```python
from build123d import *

# Parameters (mm, degrees)
SKETCH1_W                      = 15.24
SKETCH1_H                      = 15.24
BASE_FLANGE1_DEPTH             = 1.5875
EDGE_FLANGE1_STRIP_W           = 8.228
EDGE_FLANGE1_STRIP_H           = 1.5875
EDGE_FLANGE1_STRIP_CUT_DEPTH   = 15.24
EDGE_FLANGE1_STRIP_2_W         = 8.228
EDGE_FLANGE1_STRIP_2_H         = 1.5875
EDGE_FLANGE1_STRIP_CUT_2_DEPTH = 15.24
EDGE_FLANGE1_DEPTH             = 15.24
EDGE_FLANGE1_BEND_DEPTH        = 15.24
CUT_EXTRUDE2_REACH             = 30.592
CUT_EXTRUDE1_REACH             = 30.592
SKETCH13_R                     = 3.2639


# Sheet-metal steps are written as plain solids
with BuildPart() as part:
    # Sketch1 → Base-Flange1 (new body)
    with BuildSketch(Plane(origin=(0, 0, 0), x_dir=(1, 0, 0), z_dir=(0, 1, 0))):
        Rectangle(SKETCH1_W, SKETCH1_H)
    extrude(amount=-BASE_FLANGE1_DEPTH)

    # Edge-Flange1 strip (across the edge) → Edge-Flange1 strip cut (cut)
    with BuildSketch(Plane(origin=(-7.72, 0, -7.62), x_dir=(1, 0, 0), z_dir=(0, 0, 1))):
        with Locations((-3.225, -0.79375)):
            Rectangle(EDGE_FLANGE1_STRIP_W, EDGE_FLANGE1_STRIP_H)
    extrude(amount=EDGE_FLANGE1_STRIP_CUT_DEPTH, mode=Mode.SUBTRACT)

    # Edge-Flange1 strip 2 (across the edge) → Edge-Flange1 strip cut 2 (cut)
    with BuildSketch(Plane(origin=(7.72, 0, 7.62), x_dir=(-1, 0, 0), z_dir=(0, 0, -1))):
        with Locations((-3.225, -0.79375)):
            Rectangle(EDGE_FLANGE1_STRIP_2_W, EDGE_FLANGE1_STRIP_2_H)
    extrude(amount=EDGE_FLANGE1_STRIP_CUT_2_DEPTH, mode=Mode.SUBTRACT)

    # Edge-Flange1 section (across the edge) → Edge-Flange1 (add)
    with BuildSketch(Plane(origin=(-7.72, 0, -7.62), x_dir=(1, 0, 0), z_dir=(0, 0, 1))):
        with BuildLine():
            Line((-1.5875, 0.889), (-1.5875, 20.32))
            Line((-1.5875, 20.32), (0, 20.32))
            Line((0, 20.32), (0, 0.889))
            ThreePointArc((0, 0.889), (0.260382072, 0.260382072), (0.889, 0))
            Line((0.889, 0), (0.889, -1.5875))
            ThreePointArc((0.889, -1.5875), (-0.862149944, -0.862149944), (-1.5875, 0.889))
        make_face()
    extrude(amount=EDGE_FLANGE1_DEPTH)

    # Edge-Flange1 section 2 (across the edge) → Edge-Flange1 bend (add)
    with BuildSketch(Plane(origin=(7.72, 0, 7.62), x_dir=(-1, 0, 0), z_dir=(0, 0, -1))):
        with BuildLine():
            Line((-1.5875, 0.889), (-1.5875, 20.32))
            Line((-1.5875, 20.32), (0, 20.32))
            Line((0, 20.32), (0, 0.889))
            ThreePointArc((0, 0.889), (0.260382072, 0.260382072), (0.889, 0))
            Line((0.889, 0), (0.889, -1.5875))
            ThreePointArc((0.889, -1.5875), (-0.862149944, -0.862149944), (-1.5875, 0.889))
        make_face()
    extrude(amount=EDGE_FLANGE1_BEND_DEPTH)

    # Cut-Extrude2: up to this face of the body (flat: up to its plane)
    cut_extrude2_end = Plane(part.part.faces().sort_by_distance((9.3075, 10.6045, 0))[0])
    # Sketch14 → Cut-Extrude2 (cut, up to the picked face)
    with BuildSketch(Plane.ZY.offset(9.3075), mode=Mode.PRIVATE) as cut_extrude2_sk1:
        with BuildLine():
            Line((-7.62, 20.32), (-7.62, 12.7))
            ThreePointArc((-7.62, 12.7), (-5.388153673, 18.088153673), (0, 20.32))
            Line((0, 20.32), (-7.62, 20.32))
        make_face()
    cut_extrude2_tool1 = split(extrude(cut_extrude2_sk1.sketch, amount=-CUT_EXTRUDE2_REACH, mode=Mode.PRIVATE), bisect_by=cut_extrude2_end, keep=Keep.BOTH, mode=Mode.PRIVATE)
    # Sketch14 → Cut-Extrude2 (cut, up to the picked face)
    with BuildSketch(Plane.ZY.offset(9.3075), mode=Mode.PRIVATE) as cut_extrude2_sk2:
        with BuildLine():
            Line((7.62, 20.32), (0, 20.32))
            ThreePointArc((0, 20.32), (5.388153673, 18.088153673), (7.62, 12.7))
            Line((7.62, 12.7), (7.62, 20.32))
        make_face()
    cut_extrude2_tool2 = split(extrude(cut_extrude2_sk2.sketch, amount=-CUT_EXTRUDE2_REACH, mode=Mode.PRIVATE), bisect_by=cut_extrude2_end, keep=Keep.BOTH, mode=Mode.PRIVATE)
    add(cut_extrude2_tool1.solids().sort_by(Axis((-9.3075, 18.617936, -5.917936), (1, 0, 0)))[0], mode=Mode.SUBTRACT)
    add(cut_extrude2_tool2.solids().sort_by(Axis((-9.3075, 18.617936, 5.917936), (1, 0, 0)))[0], mode=Mode.SUBTRACT)

    # Cut-Extrude1: up to this face of the body (flat: up to its plane)
    cut_extrude1_end = Plane(part.part.faces().sort_by_distance((9.3075, 9.868138134, 0))[0])
    # Sketch13 → Cut-Extrude1 (cut, up to the picked face)
    with BuildSketch(Plane.ZY.offset(9.3075), mode=Mode.PRIVATE) as cut_extrude1_sk1:
        with Locations(Location((0, 12.7, 0), (0, 0, 270))):
            Circle(SKETCH13_R)
    cut_extrude1_tool1 = split(extrude(cut_extrude1_sk1.sketch, amount=-CUT_EXTRUDE1_REACH, mode=Mode.PRIVATE), bisect_by=cut_extrude1_end, keep=Keep.BOTH, mode=Mode.PRIVATE)
    add(cut_extrude1_tool1.solids().sort_by(Axis((-9.3075, 12.7, 0), (1, 0, 0)))[0], mode=Mode.SUBTRACT)


solid = part.part
```
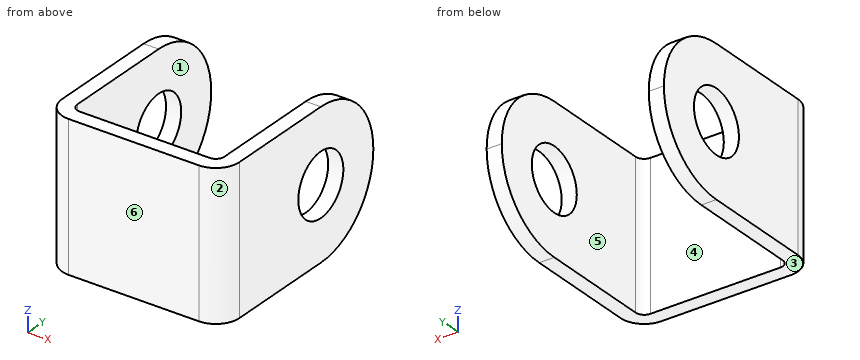
The model under review builds one solid part; all positions refer to its coordinate system, in mm. Face numbers are marked on the shaded views. A direction names the side the tool comes from. Give positions to 0.01 mm unless a question says otherwise; leave off trailing zeros. Write each loop counter-clockwise with the first axis right and the second up, starting at its lowest first coordinate (ties: lowest second). Pieces come first, ordered by that corner, then holes. Notation, with made-up numbers: M 13,16 L 28,16 A15 cw 28,30 Z; hole C 42,47 d11. An arc over 180 degrees is marked long. Write item = value, one per line. Start each with the question number.
Q1. Clearance check with flat-ended pins moving along their axes: pin 1 (5 mm diameter, centred on x = 0.5, z = -0.5, fed in from +Y); pin 2 (4 mm diameter, centred on y = 12.7, z = 0, fed in from -X); pin 3 (4 mm diameter, centred on x = -6.5, y = 8, fed in from -Z). State where each tip first meets the part, or that it passes through.
Q2. Machinability: for the marked faces 5 and 6, which of the approach directions +Z, -Z, +X, -X, +Y, -Y give a long, thin tool a straight path to every point of the face, cutting with its end or side? Answer none if there is none.
Q3. Mouldability with a two-part tool opening along X and no side actions: class the marked faces 1, 2, 3 and 4 as released by +X, released by -X, zero draft, split by the parting line, or undercut.
Q4. We need section B-B (y = 15.25). State the section outline as (x, z) points.
Q5. We need section D-D (x = 8). State the section outline as (y, z) points, plus the area to 3 significant figures.
Q6. We need section C-C (z = -5.5). State the section outline as (x, y) points, plus the area to 3 significant figures.
Q7. For line 1 (X direction, y = 11.5, z = 3.5); line 2 (Z direction, x = 8.45, y = 12.7); line 3 (Y direction, x = 5.5, z = -5.25), list the stretches that pass through material, from the lowest coordinate up.
Q8. We need section A-A (z = 2.25). State the section outline as (x, y) points.
Result set:
q1.pin_1 = 0
q1.pin_2 = through
q1.pin_3 = -7.62
q2.face_5 = +Z, -Z, +Y
q2.face_6 = +Z, -Z, +X, -X, -Y
q3.face_1 = undercut
q3.face_2 = released by +X
q3.face_3 = zero draft
q3.face_4 = undercut
q4.outline = M -9.31,-7.18 L -7.72,-7.18 L -7.72,-2.04 L -9.31,-2.04 Z; M -9.31,2.04 L -7.72,2.04 L -7.72,7.18 L -9.31,7.18 Z; M 7.72,-7.18 L 9.31,-7.18 L 9.31,-2.04 L 7.72,-2.04 Z; M 7.72,2.04 L 9.31,2.04 L 9.31,7.18 L 7.72,7.18 Z
q5.outline = M -1.29,-7.62 L 12.7,-7.62 A7.62 ccw 12.7,7.62 L -1.29,7.62 Z; hole C 12.7,0 d6.53
q5.area = 271 mm2
q6.outline = M -9.31,0.89 A2.48 ccw -6.83,-1.59 L 6.83,-1.59 A2.48 ccw 9.31,0.89 L 9.31,17.97 L 7.72,17.97 L 7.72,0.89 A0.89 cw 6.83,0 L -6.83,0 A0.89 cw -7.72,0.89 L -7.72,17.97 L -9.31,17.97 Z
q6.area = 84.3 mm2
q7.line_1 = -9.31 to -7.72, 7.72 to 9.31
q7.line_2 = -7.62 to -3.26, 3.26 to 7.62
q7.line_3 = -1.59 to 0
q8.outline = M -9.31,0.89 A2.48 ccw -6.83,-1.59 L 6.83,-1.59 A2.48 ccw 9.31,0.89 L 9.31,10.34 L 7.72,10.34 L 7.72,0.89 A0.89 cw 6.83,0 L -6.83,0 A0.89 cw -7.72,0.89 L -7.72,10.34 L -9.31,10.34 Z; M -9.31,15.06 L -7.72,15.06 L -7.72,19.98 L -9.31,19.98 Z; M 7.72,15.06 L 9.31,15.06 L 9.31,19.98 L 7.72,19.98 Z
